Could you check a few things on this model? Use its own coordinates, in mm. Face numbers are marked on the shaded views. A direction names the side the tool comes from. Coordinates: 2 decimals unless noted, no trailing zeros. Order: outer loops, then holes, each group sorted by start corner. A loop starts at its lowest first (then second) coordinate and runs counter-clockwise, first axis right, second up. Notation, with made-up numbers: (39.5, 9) - (52.5, 9) arc R16 ccw to (52.5, 15) - close; hole circle Ø10 at (-36, -16.75). An arc over 180 degrees is marked (long way). Answer as CSV lines item,"result". Start each with the question number.
1. For pin 1 (3 mm diameter, centred on x = 1.5, z = 27.5, fed in from +Y); pin 2 (1 mm diameter, centred on x = -71.5, y = 254, fed in from +Z); pin 3 (5.5 mm diameter, centred on x = 25, z = -17.5, fed in from +Y), each with a flat end and sliding along its axis, tell me the tip position at first contact or that it passes through.
2. I need wall thicknesses on probe 1 along Y at (x, z) = (64, -56.5); probe 2 along Y at (x, z) = (12.5, 12); probe 3 along X at (y, z) = (134.5, -73). Which ranges of each line are inside material? Lowest first, please.
3. I want a section at C-C, the plane x = 0. List the corners of the cut face in (y, z) for me, and give its area (3 significant figures).
4. I want a section at A-A, the plane y = 42. List the corners of the cut face in (x, z) for me, and give its area (3 significant figures).
5. I want a section at B-B, the plane y = 341.5. List the corners of the cut face in (x, z) for me, and give its area (3 significant figures).
6. For the marked faces 1, 2 and 3, which set-ups out of +Z, -Z, +X, -X, +Y, -Y let a thin tool reach every point of the face, with its end or its side?
7. I want a section at D-D, the plane y = -111.5. List the corners of the cut face in (x, z) for me, and give its area (3 significant figures).
from build123d import *

# Parameters (mm, degrees)
EXTRUDE_1_DEPTH      = 265
SKETCH_3_W           = 30.618601132
SKETCH_3_H           = 40.943060599
EXTRUDE_2_DEPTH      = 100
EXTRUDE_2_DEPTH_BACK = 153
SKETCH_5_R           = 15.723920129
EXTRUDE_3_DEPTH      = 207
EXTRUDE_3_DEPTH_BACK = 110
SKETCH_7_W           = 30.618601132
SKETCH_7_H           = 25.075478903
EXTRUDE_4_DEPTH      = 99
EXTRUDE_4_DEPTH_BACK = 153
SKETCH_8_R           = 30.618601132
EXTRUDE_5_DEPTH      = 200


with BuildPart() as part:
    # Эскиз1 → Бобышка-Вытянуть1 (new body)
    with BuildSketch(Plane(origin=(0, 0, 0), x_dir=(1, 0, 0), z_dir=(0, 1, 0))):
        Polygon((18.014188727, -24.758589212), (30.448661583, 3.22145046), (12.434472856, 27.980039673), (-18.014188727, 24.758589212), (-30.448661583, -3.22145046), (-12.434472856, -27.980039673), align=None)
    extrude(amount=EXTRUDE_1_DEPTH)

    # Эскиз3 → Бобышка-Вытянуть2 (add, two sides)
    with BuildSketch(Plane(origin=(21.44156722, 0, -15.600745066), x_dir=(-0.588341337, 0, -0.808612683), z_dir=(0.808612683, 0, -0.588341337))) as extrude_2_sk:
        with Locations((0, 244.89483014)):
            Rectangle(SKETCH_3_W, SKETCH_3_H)
    extrude(amount=EXTRUDE_2_DEPTH)
    extrude(extrude_2_sk.sketch, amount=-EXTRUDE_2_DEPTH_BACK)

    # Эскиз5 → Бобышка-Вытянуть3 (add, two sides)
    with BuildSketch(Plane(origin=(0, 265.366360439, 0), x_dir=(1, 0, 0), z_dir=(0, 1, 0))) as extrude_3_sk:
        with Locations((-89.323031668, -64.478103556)):
            Circle(SKETCH_5_R)
        with Locations((88.86181825, 65.168036102)):
            Circle(SKETCH_5_R)
    extrude(amount=EXTRUDE_3_DEPTH)
    extrude(extrude_3_sk.sketch, amount=-EXTRUDE_3_DEPTH_BACK)

    # Эскиз7 → Бобышка-Вытянуть4 (add, two sides)
    with BuildSketch(Plane(origin=(21.44156722, 0, -15.600745066), x_dir=(-0.588341337, 0, -0.808612683), z_dir=(0.808612683, 0, -0.588341337))) as extrude_4_sk:
        with Locations((0, 141.302670342)):
            Rectangle(SKETCH_7_W, SKETCH_7_H)
    extrude(amount=EXTRUDE_4_DEPTH)
    extrude(extrude_4_sk.sketch, amount=-EXTRUDE_4_DEPTH_BACK)

    # Эскиз8 → Бобышка-Вытянуть5 (add)
    with BuildSketch(Plane.XZ):
        Circle(SKETCH_8_R)
    extrude(amount=EXTRUDE_5_DEPTH)


solid = part.part
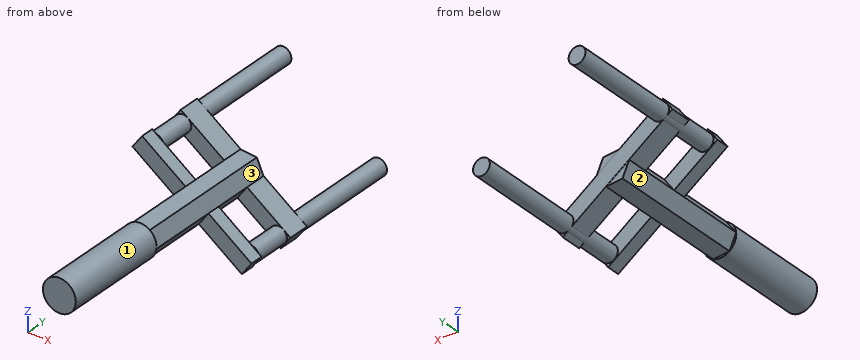
Solved:
1,pin 1,"stops at y = 265"
1,pin 2,"stops at z = 71.32"
1,pin 3,"stops at y = 265.37"
2,probe 1,"y = 128.76 to 153.84, 224.42 to 265.37"
2,probe 2,"y = -200 to 265"
2,probe 3,"x = 74.31 to 102.11"
3,outline,"(-200, -30.62) - (0, -30.62) - (0, -26.66) - (265, -26.66) - (265, -18.93) - (265.37, -18.93) - (265.37, 18.93) - (265, 18.93) - (265, 26.66) - (0, 26.66) - (0, 30.62) - (-200, 30.62) - close"
3,area,"26,400 mm2"
4,outline,"(-30.45, 3.22) - (-18.01, -24.76) - (12.43, -27.98) - (30.45, -3.22) - (18.01, 24.76) - (-12.43, 27.98) - close"
4,area,"2,440 mm2"
5,outline,"circle Ø31.45 at (-89.32, 64.48); circle Ø31.45 at (88.86, -65.17)"
5,area,"1,550 mm2"
6,face 1,"-Y"
6,face 2,"-Z, -X, +Y"
6,face 3,"+Z, +X, +Y"
7,outline,"circle Ø61.24 at (0, 0)"
7,area,"2,950 mm2"
